Input: part model. Units: mm. Frame: model coordinates. Face numbers are marked on the shaded views. A direction names the side the tool comes from. Round coordinates to 2 decimals unless told otherwise and drop trailing zeros. Order: outer loops, then holes, each group sorted by start corner. A loop starts at its lowest first (then second) coordinate and runs counter-clockwise, first axis right, second up. Notation, with made-up numbers: (83, -3.75) -> (90, -3.75) arc R15 ccw to (90, 6.25) -> close; hole circle Ø1 at (25.5, -2). An arc over 180 degrees is marked (long way). Use a Markdown table: item, result.
from build123d import *

# Parameters (mm, degrees)
F1_DEPTH      = 1
F3_DEPTH      = 25
F6_DEPTH      = 5
F6_DEPTH_BACK = 5
F8_W          = 12
F8_H          = 1
F9_DEPTH      = 20
F10_T1_DEPTH  = 13.0901699437
F10_T3_DEPTH  = 15
F10_T5_DEPTH  = 11.1803398875


# Not quite as in the source:
# - a fillet or chamfer that OpenCascade refuses, or shapes differently, is made with other operations: its cross-section is extruded or revolved along the edge and cut away or added


with BuildPart() as f1:
    # F0 (on Top) → F1 (new body)
    with BuildSketch(Plane.XY):
        Polygon((0, 50), (0, 0), (50, 0), (50, 50), (31, 50), (31, 35), (30, 35), (30, 60), (20, 60), (20, 35), (19, 35), (19, 50), align=None)
    extrude(amount=F1_DEPTH)

    # F2 (on Top) → F3 (join)
    with BuildSketch(Plane.XY):
        Polygon((0, 50), (0, 0), (50, 0), (50, 50), (31, 50), (31, 49), (49, 49), (49, 1), (1, 1), (1, 49), (19, 49), (19, 50), align=None)
    extrude(amount=F3_DEPTH)

    # F5 (on offset) → F6 (join, two sides)
    with BuildSketch(Plane.YZ.offset(25)) as f6_sk:
        Polygon((57.5, -5), (60, 0), (55, 0), (55, -5), align=None)
    extrude(amount=F6_DEPTH)
    extrude(f6_sk.sketch, amount=-F6_DEPTH_BACK)

    # F8 (on offset) → F9 (join)
    with BuildSketch(Plane.XY.offset(25)):
        with Locations((25, 49.5)):
            Rectangle(F8_W, F8_H)
    extrude(amount=-F9_DEPTH)

    # F10: fillet of radius 1 on 4 edges, made by hand

    # F10_s2 → F10_t1 (cut)
    with BuildSketch(Plane.YZ.offset(18.4549150281)):
        with BuildLine():
            ThreePointArc((57.7763932023, -4.4472135955), (57.4076971234, -4.8506508084), (56.8819660113, -5))
            Line((56.8819660113, -5), (57.5, -5))
            Line((57.5, -5), (57.7763932023, -4.4472135955))
        make_face()
    extrude(amount=F10_T1_DEPTH, mode=Mode.SUBTRACT)

    # F10_s4 → F10_t3 (cut)
    with BuildSketch(Plane.YZ.offset(17.5)):
        with BuildLine():
            ThreePointArc((56, -5), (55.2928932188, -4.7071067812), (55, -4))
            Line((55, -4), (55, -5))
            Line((55, -5), (56, -5))
        make_face()
        with BuildLine():
            ThreePointArc((59, 1), (59.7071067812, 0.7071067812), (60, 0))
            Line((60, 0), (60, 1))
            Line((60, 1), (59, 1))
        make_face()
    extrude(amount=F10_T3_DEPTH, mode=Mode.SUBTRACT)

    # F10_s6 → F10_t5 (cut)
    with BuildSketch(Plane.YZ.offset(19.4098300563)):
        with BuildLine():
            ThreePointArc((60, 0.2360679775), (59.9732489895, 0.006315057), (59.894427191, -0.211145618))
            Line((59.894427191, -0.211145618), (60, 0))
            Line((60, 0), (60, 0.2360679775))
        make_face()
    extrude(amount=F10_T5_DEPTH, mode=Mode.SUBTRACT)


solid = f1.part
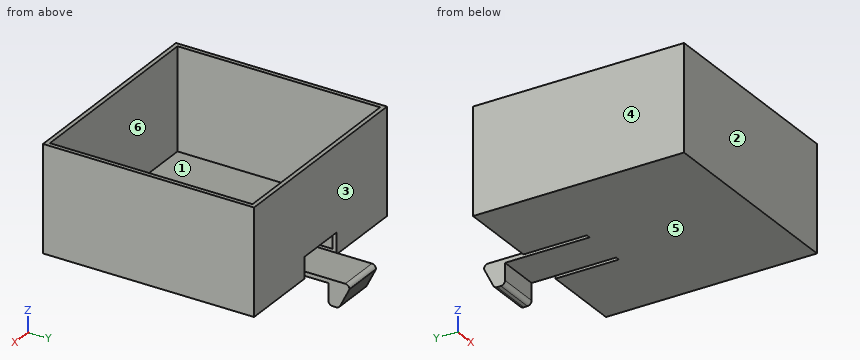
1) Line query: L1, parallel to X at y = 41, z = 5; L2, parallel to Z at x = 22, y = 48. Output: solid intervals per line, ascending. Write a range as [from, to].
Results found:
| item | result |
|---|---|
| L1 | x = [0, 1], [49, 50] |
| L2 | z = [0, 1] |
2) Pull-direction query (Y, two-part tool) for the marked faces 1, 2 and 3; classes: +Y half, -Y half, draft (parallel to the pull), parting line (faces both ways), or undercut.
Results found:
| item | result |
|---|---|
| face 1 | undercut |
| face 2 | -Y half |
| face 3 | +Y half |
3) Pin query (flat end, axial travel): pin 1 Ø12.5 at (x, z) = (31, 14.5) entering from +Y; pin 2 Ø3 at (x, y) = (5, 37.5) entering from +Z; pin 3 Ø1.5 at (x, y) = (32, 35.5) entering from -Z. Return the tip coordinate at first contact, or that it passes through.
Results found:
| item | result |
|---|---|
| pin 1 | stops at y = 50 |
| pin 2 | stops at z = 1 |
| pin 3 | stops at z = 0 |
4) Cut plane A-A on y = 37.5. Return loops of the section in (x, z), and give its area (3 significant figures).
Results found:
| item | result |
|---|---|
| outline | (0, 0) -> (19, 0) -> (19, 1) -> (1, 1) -> (1, 25) -> (0, 25) -> close; (20, 0) -> (30, 0) -> (30, 1) -> (20, 1) -> close; (31, 0) -> (50, 0) -> (50, 25) -> (49, 25) -> (49, 1) -> (31, 1) -> close |
| area | 96.0 mm² |
5) Cut plane D-D on y = 19. Return loops of the section in (x, z), and give its area (3 significant figures).
Results found:
| item | result |
|---|---|
| outline | (0, 0) -> (50, 0) -> (50, 25) -> (49, 25) -> (49, 1) -> (1, 1) -> (1, 25) -> (0, 25) -> close |
| area | 98.0 mm² |
6) Cut plane B-B on x = 23. Return loops of the section in (y, z), and give its area (3 significant figures).
Results found:
| item | result |
|---|---|
| outline | (0, 0) -> (55, 0) -> (55, -4) arc R1 ccw to (56, -5) -> (56.88, -5) arc R1 ccw to (57.78, -4.45) -> (59.89, -0.21) arc R1 ccw to (59.99, 0.12) arc R1 ccw to (59, 1) -> (1, 1) -> (1, 25) -> (0, 25) -> close; (49, 5) -> (50, 5) -> (50, 25) -> (49, 25) -> close |
| area | 122 mm² |
7) Set-up query: the marked faces 4, 5 and 6. Return all of +Z, -Z, +X, -X, +Y, -Y with unobstructed straight access to the full face (end or side cutting, diameter ignored); none if empty.
Results found:
| item | result |
|---|---|
| face 4 | +Z, -Z, -X, +Y, -Y |
| face 5 | -Z, +X, -X, -Y |
| face 6 | +Z |
8) Cut plane C-C on z = 12.5. Return loops of the section in (x, y), and give its area (3 significant figures).
Results found:
| item | result |
|---|---|
| outline | (0, 0) -> (50, 0) -> (50, 50) -> (0, 50) -> close; hole (1, 1) -> (49, 1) -> (49, 49) -> (1, 49) -> close |
| area | 196 mm² |
